Autodesk Inventor part; units mm, degrees
ref_plane "YZ Plane" through (0, 0, 0) normal (1, 0, 0) x (0, 1, 0)
ref_plane "XZ Plane" through (0, 0, 0) normal (0, 1, 0) x (-1, 0, 0)
ref_plane "XY Plane" through (0, 0, 0) normal (0, 0, 1) x (1, 0, 0)
sketch "Boceto1" plane through (0, 0, 0) normal (0, 0, 1) x (1, 0, 0)
  line L0 (-80, -80) -> (80, -80)
  line L1 (80, -80) -> (80, 80)
  line L2 (80, 80) -> (-80, 80)
  line L3 (-80, 80) -> (-80, -80)
  line L4 (-80, -80) -> (80, 80) construction
  line L5 (80, -80) -> (-80, 80) construction
  circle A0 centre (0, -14.988) radius 12.5
  circle A1 centre (0, 18) radius 2.5
  point P0 (0, 0)
  dimension "d0" = 160
  dimension "d1" = 160
  dimension "d2" = 25
  dimension "d3" = 14.988
  dimension "d4" = 5
  dimension "d5" = 18
extrude "Extrusión1" add sketch "Boceto1" along normal blind 10
sketch "Boceto2" plane through (0, 0, 0) normal (0, 0, -1) x (-1, 0, 0)
  line L0 (80, 80) -> (80, -80)
  line L1 (-80, 80) -> (80, 80)
  line L2 (-80, -80) -> (-80, 80)
  line L3 (80, -80) -> (-80, -80)
  line L4 (-80, -80) -> (-80, 80) construction
  line L5 (-80, 0) -> (80, 0) construction
  line L6 (0, -80) -> (0, 80) construction
  line L7 (-80, 80) -> (80, 80) construction
  point P0 (0, 0)
  point P1 (75, 50)
  point P2 (75, -50)
  point P3 (50, -75)
  point P4 (-50, -75)
  point P5 (-75, 50)
  point P6 (-75, -50)
  dimension "d20" = 30
  dimension "d21" = 30
hole "Agujero1" at (-75, 50, 0) at (-75, -50, 0) at (-50, -75, 0) at (50, -75, 0) at (75, -50, 0) at (75, 50, 0) direction (0, 0, 1) diameter 5.5 depth 20 tip angle 118 countersink diameter 11 countersink angle 90
sketch "Boceto3" plane through (0, 0, 0) normal (0, 0, -1) x (-1, 0, 0)
  circle A0 centre (0, -14.988) radius 12.5
  circle A1 centre (0, 18) radius 2.5
  arc A2 (8.0623, 18) -> (-8.0623, 18) centre (0, 18) ccw
  arc A3 (-8.0623, 0.8759) -> (8.0623, 0.8759) centre (0, -14.988) ccw
  line L0 (-8.0623, 18) -> (-8.0623, 0.8759)
  line L1 (8.0623, 18) -> (8.0623, 0.8759)
  point P0 (0, 0)
  dimension "d22" = 5.5623
  dimension "d23" = 5.2951
extrude "Extrusión2" cut sketch "Boceto3" against normal blind 5
properties part number "TAPA TRASERA" material "Plástico PMMA"
Source: CAD feature listing. Evaluate the final solid. Frame: model axes, mm. A direction names the side the tool comes from. Coordinates: 2 decimals unless noted, no trailing zeros. Loops run counter-clockwise (first coordinate to the right, second up) from the corner with the lowest first, then second, coordinate; pieces in that order, holes last. Notation, with made-up numbers: M 11,8 L 63,8 A13 ccw 63,26 Z; hole C 59.5,48 d11. An arc over 180 degrees is marked long. Use CSV: the item, a comma, the result in double quotes.
(1) Cut plane A-A on x = 75. Return loops of the section in (y, z), and give its area (3 significant figures).
Answers follow:
outline,"M -80,0 L -55.5,0 L -52.75,2.75 L -52.75,10 L -80,10 Z; M -47.25,2.75 L -44.5,0 L 44.5,0 L 47.25,2.75 L 47.25,10 L -47.25,10 Z; M 52.75,2.75 L 55.5,0 L 80,0 L 80,10 L 52.75,10 Z"
area,"1,470 mm²"
(2) Cut plane B-B on y = -6.5. Return loops of the section in (x, z).
Answers follow:
outline,"M -80,0 L -15.64,0 L -15.64,5 L -9.18,5 L -9.18,10 L -80,10 Z; M 9.18,5 L 15.64,5 L 15.64,0 L 80,0 L 80,10 L 9.18,10 Z"
(3) Contact query for flat-ended pins moving along their axis: pin 1 (6.5 mm diameter, centred on x = 75, y = 50, fed in from -Z); pin 2 (9 mm diameter, centred on x = -75, y = 50, fed in from -Z); pin 3 (5 mm diameter, centred on x = -75, y = -50, fed in from -Z). Output: stop coordinate, or through.
Answers follow:
pin 1,"z = 2.25"
pin 2,"z = 1"
pin 3,"through"
(4) Draft query along Y for faces 1 (the face through (-1, -80, 5)), 2 (the face through (72.41, -48.65, 2.58)), 3 (the face through (-51.859, -77.027, 6.426)), 4 (the face through (-19, 1, 0)). Return one class per face: pulls with the +Y half, pulls with the -Y half, needs draft (parallel to the pull), parting line crosses it, or undercut.
Answers follow:
face 1,"pulls with the -Y half"
face 2,"undercut"
face 3,"undercut"
face 4,"needs draft"
(5) Cut plane C-C on x = -50. Return loops of the section in (y, z), and give its area (3 significant figures).
Answers follow:
outline,"M -80,0.5 L -77.75,2.75 L -77.75,10 L -80,10 Z; M -72.25,2.75 L -69.5,0 L 80,0 L 80,10 L -72.25,10 Z"
area,"1,540 mm²"
(6) Reachability of faces 5 (the face through (4.2, -2.9, 5)), 6 (the face through (80, -1, 5)) from +Z, -Z, +X, -X, +Y, -Y: full face, straight path, thin tool, end or side. Return the list, or none.
Answers follow:
face 5,"-Z"
face 6,"+Z, -Z, +X, +Y, -Y"
(7) Line query: line 1 (Y direction, x = 75, z = 5); line 2 (Y direction, x = 0, z = 7.9); line 3 (X direction, y = 50, z = 7). Output: solid intervals per line, ascending. Write a range as [from, to].
Answers follow:
line 1,"[-80, -52.75], [-47.25, 47.25], [52.75, 80]"
line 2,"[-80, -27.49], [-2.49, 15.5], [20.5, 80]"
line 3,"[-80, -77.75], [-72.25, 72.25], [77.75, 80]"
(8) Cut plane D-D on y = 50. Return loops of the section in (x, z).
Answers follow:
outline,"M -80,0.5 L -77.75,2.75 L -77.75,10 L -80,10 Z; M -72.25,2.75 L -69.5,0 L 69.5,0 L 72.25,2.75 L 72.25,10 L -72.25,10 Z; M 77.75,2.75 L 80,0.5 L 80,10 L 77.75,10 Z"
